Here's how the part is built. I have some questions about the finished solid (model axes, mm). A direction names the side the tool comes from. Coordinates: 2 decimals unless noted, no trailing zeros. Order: outer loops, then holes, each group sorted by start corner. A loop starts at its lowest first (then second) coordinate and runs counter-clockwise, first axis right, second up. Notation, with made-up numbers: (50, -30.75) - (87, -30.75) arc R22 ccw to (87, 8.25) - close; hole circle Ø9 at (51, 18). An arc over 180 degrees is marked (long way). Answer as CSV lines item,"result". Start each with the question number.
Item 1: Imagine slicing it at D-D on x = 17. List the corners of the cut face in (y, z) for me, and give its area (3 significant figures).
Item 2: Imagine slicing it at B-B on y = -69.5. List the corners of the cut face in (x, z) for me, and give its area (4 significant figures).
Item 3: On a 3-axis mill with a long thin cutter (end or side, diameter ignored), from which of +Z, -Z, +X, -X, +Y, -Y can I reach the whole of each face in a straight line? I mean faces 1 (the face through (-7.3, -47.3, 24.138)), 2 (the face through (-56.667, 3.913, 65.895)), 3 (the face through (-55, 4, 24.138)). Say none if no direction works.
Item 4: Imagine slicing it at A-A on x = 45. List the corners of the cut face in (y, z) for me, and give its area (3 significant figures).
Item 5: We'd pull the mould along X, two halves only. Please class faces 4 (the face through (-35, -45, 20)), 5 (the face through (-0.15, -88.03, 20.22)), 6 (the face through (75, 4, 65)), 7 (the face through (1, 7.938, 51)): pulls with the +X half, pulls with the -X half, needs draft (parallel to the pull), parting line crosses it, or undercut.
Item 6: I need wall thicknesses on line 1 (Y direction, x = 11, z = 57); line 2 (Z direction, x = 45.5, y = 4.5); line 3 (Z direction, x = -12, y = -10). Which ranges of each line are inside material? Lowest first, please.
Item 7: I'm going to push flat-ended pins straight in: pin 1 (21 mm diameter, centred on x = -14.5, y = -50, fed in from +Z); pin 2 (4 mm diameter, centred on y = -52, z = 20.5, fed in from +X); pin 3 (6.5 mm diameter, centred on x = -58.5, y = 3.5, fed in from -Z). Where does each tip first touch, or does it pass through?
Item 8: Imagine slicing it at C-C on x = 0. List the corners of the cut face in (y, z) for me, and give its area (3 significant figures).
from build123d import *

# Parameters (mm, degrees)
CROQUIS1_R                 = 6.35
CROQUIS1_R_2               = 6.26
CROQUIS1_R_3               = 6.25
SALIENTE_EXTRUIR1_DEPTH    = 7.9375
CROQUIS2_W                 = 150
CROQUIS2_H                 = 104.1375
SALIENTE_EXTRUIR2_DEPTH    = 7.9375
CONVERTIR_S_LIDO4_START    = -75
CONVERTIR_S_LIDO4_DEPTH    = 150
CONVERTIR_S_LIDO4_2_DEPTH  = 150
CORTAR_EXTRUIR4_DEPTH      = 369.571050011
CORTAR_EXTRUIR4_DEPTH_BACK = 369.571050011
CROQUIS4_W                 = 150
CROQUIS4_H                 = 11.2
CROQUIS7_W                 = 70
CROQUIS7_H                 = 96.03125
CROQUIS7_H_2               = 7.9375
SALIENTE_EXTRUIR3_DEPTH    = 7.9375


# Read off the part's stored shape, not the designer's step: Convertir-Sólido4
with BuildPart() as part:
    # Croquis1 → Saliente-Extruir1 (new body)
    with BuildSketch(Plane.XY):
        with BuildLine():
            Line((-75, 16), (-75, 0))
            Line((-75, 0), (75, 0))
            Line((75, 0), (75, 54))
            ThreePointArc((75, 54), (60.355339059, 89.355339059), (25, 104))
            Line((25, 104), (-200, 104))
            ThreePointArc((-200, 104), (-235.355339059, 89.355339059), (-250, 54))
            Line((-250, 54), (-250, 0))
            ThreePointArc((-250, 0), (0, -250), (250, 0))
            ThreePointArc((250, 0), (200, 50), (150, 0))
            ThreePointArc((150, 0), (0, -150), (-150, 0))
            Line((-150, 0), (-150, 16))
            Line((-150, 16), (-75, 16))
        make_face()
        with BuildLine():
            ThreePointArc((-49.374105038, 47.65), (-55.724105038, 54), (-49.374105038, 60.35))
            Line((-49.374105038, 60.35), (49.374105038, 60.35))
            ThreePointArc((49.374105038, 60.35), (55.724105038, 54), (49.374105038, 47.65))
            Line((49.374105038, 47.65), (-49.374105038, 47.65))
        make_face(mode=Mode.SUBTRACT)
        with Locations((193.418858597, -50.883643138)):
            Circle(CROQUIS1_R, mode=Mode.SUBTRACT)
        with Locations((200, 0)):
            Circle(CROQUIS1_R_2, mode=Mode.SUBTRACT)
        with Locations((-100, -173.205080757)):
            Circle(CROQUIS1_R_3, mode=Mode.SUBTRACT)
        with Locations((-50.883643138, -193.418858597)):
            Circle(CROQUIS1_R, mode=Mode.SUBTRACT)
        with Locations((-140.775956893, -142.063823547)):
            Circle(CROQUIS1_R, mode=Mode.SUBTRACT)
        with Locations((-173.205080757, -100)):
            Circle(CROQUIS1_R, mode=Mode.SUBTRACT)
        with Locations((0, -200)):
            Circle(CROQUIS1_R_3, mode=Mode.SUBTRACT)
        with Locations((52.642901704, -192.947466685)):
            Circle(CROQUIS1_R, mode=Mode.SUBTRACT)
        with Locations((100, -173.205080757)):
            Circle(CROQUIS1_R_3, mode=Mode.SUBTRACT)
        with Locations((142.063823547, -140.775956893)):
            Circle(CROQUIS1_R, mode=Mode.SUBTRACT)
        with Locations((173.205080757, -100)):
            Circle(CROQUIS1_R_3, mode=Mode.SUBTRACT)
        with Locations((-192.947466685, -52.642901704)):
            Circle(CROQUIS1_R, mode=Mode.SUBTRACT)
        with Locations((-200, 0)):
            Circle(CROQUIS1_R, mode=Mode.SUBTRACT)
        with Locations((-200, 54)):
            Circle(CROQUIS1_R, mode=Mode.SUBTRACT)
    extrude(amount=SALIENTE_EXTRUIR1_DEPTH)

    # Croquis2 → Saliente-Extruir2 (add)
    with BuildSketch(Plane.XZ):
        with Locations((0, 52.06875)):
            Rectangle(CROQUIS2_W, CROQUIS2_H)
        with BuildLine():
            Line((-50.16849794, 72.5375), (50.16849794, 72.5375))
            ThreePointArc((50.16849794, 72.5375), (56.66849794, 66.0375), (50.16849794, 59.5375))
            Line((50.16849794, 59.5375), (-50.16849794, 59.5375))
            ThreePointArc((-50.16849794, 59.5375), (-56.66849794, 66.0375), (-50.16849794, 72.5375))
        make_face(mode=Mode.SUBTRACT)
    extrude(amount=-SALIENTE_EXTRUIR2_DEPTH)

    # Convertir-Sólido4 outline → Convertir-Sólido4 (cut)
    with BuildSketch(Plane.YZ.offset(CONVERTIR_S_LIDO4_START)):
        with BuildLine():
            Line((0, 12.9375), (0, 0))
            Line((0, 0), (12.9375, 0))
            ThreePointArc((12.9375, 0), (3.789306018, 3.789306018), (0, 12.9375))
        make_face()
    extrude(amount=CONVERTIR_S_LIDO4_DEPTH, mode=Mode.SUBTRACT)

    # Convertir-S_lido4 2 outline → Convertir-S_lido4 2 (add)
    with BuildSketch(Plane.YZ.offset(CONVERTIR_S_LIDO4_START)):
        with BuildLine():
            Line((7.9375, 12.9375), (7.9375, 7.9375))
            Line((7.9375, 7.9375), (12.9375, 7.9375))
            ThreePointArc((12.9375, 7.9375), (9.401966094, 9.401966094), (7.9375, 12.9375))
        make_face()
    extrude(amount=CONVERTIR_S_LIDO4_2_DEPTH)

    # Croquis4 → Cortar-Extruir4 (cut, two sides: drawn at the far end of the back side and taken through both)
    with BuildSketch(Plane.XZ.offset(-CORTAR_EXTRUIR4_DEPTH_BACK)):
        Polygon((-75, 12.9375), (-75, 24.1375), (-279.933014074, 24.1375), (-279.933014074, -40.537488795), (278.241575923, -40.537488795), (278.241575923, 24.1375), (75, 24.1375), (75, 12.9375), align=None)
        with Locations((0, 18.5375)):
            Rectangle(CROQUIS4_W, CROQUIS4_H)
    extrude(amount=CORTAR_EXTRUIR4_DEPTH + CORTAR_EXTRUIR4_DEPTH_BACK, mode=Mode.SUBTRACT)

    # Croquis7 → Saliente-Extruir3 (add)
    # profile 1 of 2: a face of its own
    with BuildSketch(Plane(origin=(0, 0, 24.1375), x_dir=(-1, 0, 0), z_dir=(0, 0, -1))):
        with Locations((0, -48.015625)):
            Rectangle(CROQUIS7_W, CROQUIS7_H)
        with BuildLine():
            ThreePointArc((-7, -13.240738452), (0, -6.240738452), (7, -13.240738452))
            Line((7, -13.240738452), (7, -81.03125))
            ThreePointArc((7, -81.03125), (0, -88.03125), (-7, -81.03125))
            Line((-7, -81.03125), (-7, -13.240738452))
        make_face(mode=Mode.SUBTRACT)
    # profile 2 of 2: a face of its own
    with BuildSketch(Plane(origin=(0, 0, 24.1375), x_dir=(-1, 0, 0), z_dir=(0, 0, -1))):
        with Locations((0, 3.96875)):
            Rectangle(CROQUIS7_W, CROQUIS7_H_2)
    extrude(amount=SALIENTE_EXTRUIR3_DEPTH)


solid = part.part
Responses:
1,outline,"(-96.03, 16.2) - (7.94, 16.2) - (7.94, 59.54) - (0, 59.54) - (0, 24.14) - (-96.03, 24.14) - close; (0, 72.54) - (7.94, 72.54) - (7.94, 104.14) - (0, 104.14) - close"
1,area,"1,360 mm^2"
2,outline,"(-35, 16.2) - (-7, 16.2) - (-7, 24.14) - (-35, 24.14) - close; (7, 16.2) - (35, 16.2) - (35, 24.14) - (7, 24.14) - close"
2,area,"444.5 mm^2"
3,face 1,"+Z, +X, -X, -Y"
3,face 2,"+Y, -Y"
3,face 3,"-Z, -X, +Y, -Y"
4,outline,"(0, 24.14) - (7.94, 24.14) - (7.94, 59.54) - (0, 59.54) - close; (0, 72.54) - (7.94, 72.54) - (7.94, 104.14) - (0, 104.14) - close"
4,area,"532 mm^2"
5,face 4,"pulls with the -X half"
5,face 5,"undercut"
5,face 6,"pulls with the +X half"
5,face 7,"needs draft"
6,line 1,"y = 0 to 7.94"
6,line 2,"z = 24.14 to 59.54, 72.54 to 104.14"
6,line 3,"z = 16.2 to 24.14"
7,pin 1,"stops at z = 24.14"
7,pin 2,"stops at x = 35"
7,pin 3,"stops at z = 24.14"
8,outline,"(-96.03, 16.2) - (-88.03, 16.2) - (-88.03, 24.14) - (-96.03, 24.14) - close; (-6.24, 16.2) - (7.94, 16.2) - (7.94, 59.54) - (0, 59.54) - (0, 24.14) - (-6.24, 24.14) - close; (0, 72.54) - (7.94, 72.54) - (7.94, 104.14) - (0, 104.14) - close"
8,area,"708 mm^2"
